CAD build for the part. Positions are in the model's coordinates, mm. Face numbers are marked on the shaded views. A direction names the side the tool comes from. Coordinates: 2 decimals unless noted, no trailing zeros. Write each loop counter-clockwise with the first axis right and the second up, starting at its lowest first coordinate (ties: lowest second). Pieces come first, ordered by that corner, then holes. Notation, with made-up numbers: M -1.5,68 L 27.5,68 A19 cw 27.5,99 Z; hole C 39,-16 d3. An arc over 180 degrees is marked long. Answer as CSV lines item,"result". Start each with the question number.
Autodesk Inventor part; units mm, degrees
ref_plane "to_bearing_XY" through (0, 0, -4) normal (0, 0, -1) x (1, 0, 0)
ref_plane "to_bearing_YZ" through (0, 0, -4) normal (1, 0, 0) x (0, -1, 0)
ref_plane "to_bearing_ZX" through (0, 0, -4) normal (0, -1, 0) x (0, 0, -1)
sketch "_____1" plane through (0, 0, 0) normal (0, 0, 1) x (1, 0, 0)
  line L0 (-16, 15) -> (-16, -25)
  line L1 (-16, -25) -> (16, -25)
  line L2 (16, -25) -> (16, 15)
  line L3 (16, 15) -> (-16, 15)
extrude "Extrusion1" add sketch "_____1" along normal mid plane 12
sketch "Sketch_2" plane through (0, 0, 0) normal (1, 0, 0) x (0, 1, 0)
  line L0 (0, -6) -> (0, 6)
  line L1 (0, 6) -> (11, 6)
  line L2 (11, 6) -> (11, 3.15)
  line L3 (11, 3.15) -> (11.5, 3.15)
  line L4 (11.5, 3.15) -> (11.5, 2)
  line L5 (11.5, 2) -> (11, 2)
  line L6 (11, 2) -> (11, -4)
  line L7 (11, -4) -> (9.5, -4)
  line L8 (9.5, -4) -> (9.5, -6)
  line L9 (9.5, -6) -> (0, -6)
  line L10 (0, -6) -> (0, 6)
revolve "Revolution1" cut sketch "Sketch_2" angle 360 about axis through (0, 0, -6) along (0, 0, -1)
sketch "Sketch3" plane through (-16, -25, 6) normal (0, -1, 0) x (1, 0, 0)
  point P0 (6, -6)
hole "Hole1" at (-10, -25, 0) direction (0, 1, 0) diameter 4.134 depth 10 tip angle 120 countersink diameter 5 countersink angle 90
pattern_linear "Rectangular Pattern1" count 2 spacing 20 along (1, 0, 0) of "Hole1"
ref_plane "to_bearing_XY" through (0, 0, -4) normal (0, 0, -1) x (1, 0, 0)
ref_plane "to_bearing_YZ" through (0, 0, -4) normal (1, 0, 0) x (0, -1, 0)
ref_plane "to_bearing_ZX" through (0, 0, -4) normal (0, -1, 0) x (0, 0, -1)
ref_plane "to_ring_XY" through (0, 0, 2) normal (0, 0, -1) x (1, 0, 0)
ref_plane "to_ring_YZ" through (0, 0, 2) normal (1, 0, 0) x (0, -1, 0)
ref_plane "to_ring_ZX" through (0, 0, 2) normal (0, -1, 0) x (0, 0, -1)
properties part number "BGBFS6900DD-25-_h"
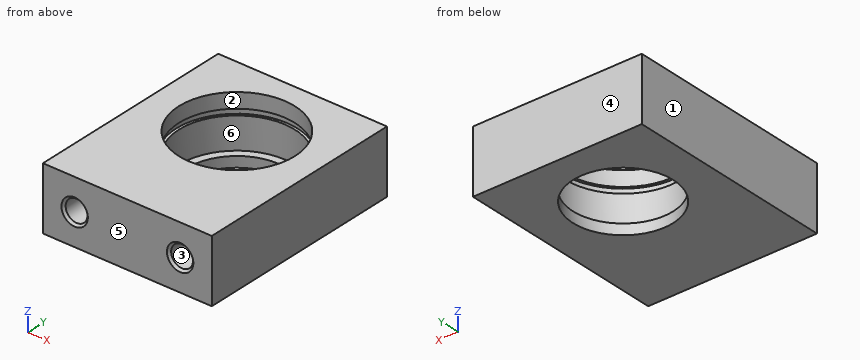
1) Probe L1, parallel to X at y = -20, z = 0; L2, parallel to X at y = 0, z = -5.45; L3, parallel to Z at x = 11, y = -1.5. List the from-to ranges inside material, lowest first. Write a range as [from, to].
2) Band-saw the part on D-D, the plane z = -3.25. List the corners of the cut face in (x, y), plus the area to 3 significant figures.
3) Two-plate mould, pull along Y, no slides. Class the marked faces 4, 5 and 6: pulls with the +Y half, pulls with the -Y half, needs draft (parallel to the pull), parting line crosses it, or undercut.
4) Band-saw the part on B-B, the plane x = 0. List the corners of the cut face in (y, z).
5) Band-saw the part on C-C, the plane y = -22. List the corners of the cut face in (x, z).
6) Pin check, flat tip, straight feed: P1, Ø11, axis at x = 1, y = -4.5, coming from the +Z side. Stop position of the tip, or through.
7) Band-saw the part on A-A, the plane y = 0. List the corners of the cut face in (x, z), plus the area to 3 significant figures.
8) Tool access for the marked faces 1, 2 and 3: list every direction of +Z, -Z, +X, -X, +Y, -Y with a clear straight run to the whole face (end or side of a thin tool).
Result sheet:
1,L1,"x = [-16, -12.07], [-7.93, 7.93], [12.07, 16]"
1,L2,"x = [-16, -9.5], [9.5, 16]"
1,L3,"z = [-6, 2], [3.15, 6]"
2,outline,"M -16,-25 L 16,-25 L 16,15 L -16,15 Z; hole C 0,0 d22"
2,area,"900 mm²"
3,face 4,"pulls with the +Y half"
3,face 5,"pulls with the -Y half"
3,face 6,"undercut"
4,outline,"M -25,-6 L -9.5,-6 L -9.5,-4 L -11,-4 L -11,2 L -11.5,2 L -11.5,3.15 L -11,3.15 L -11,6 L -25,6 Z; M 9.5,-6 L 15,-6 L 15,6 L 11,6 L 11,3.15 L 11.5,3.15 L 11.5,2 L 11,2 L 11,-4 L 9.5,-4 Z"
5,outline,"M -16,-6 L 16,-6 L 16,6 L -16,6 Z; hole C -10,0 d4.13; hole C 10,0 d4.13"
6,P1,"stops at z = -4"
7,outline,"M -16,-6 L -9.5,-6 L -9.5,-4 L -11,-4 L -11,2 L -11.5,2 L -11.5,3.15 L -11,3.15 L -11,6 L -16,6 Z; M 9.5,-6 L 16,-6 L 16,6 L 11,6 L 11,3.15 L 11.5,3.15 L 11.5,2 L 11,2 L 11,-4 L 9.5,-4 Z"
7,area,"125 mm²"
8,face 1,"+Z, -Z, -X, +Y, -Y"
8,face 2,"+Z"
8,face 3,"-Y"
